Verification items for the finished model (mm, model axes). A direction names the side the tool comes from. Round coordinates to 2 decimals unless told otherwise and drop trailing zeros. Loops run counter-clockwise (first coordinate to the right, second up) from the corner with the lowest first, then second, coordinate; pieces in that order, holes last. Notation, with made-up numbers: M 69,-9 L 80,-9 A13 cw 80,14 Z; hole C 14,58 d11. An arc over 180 degrees is marked long. One line per item, written item: value.
from build123d import *

# Parameters (mm, degrees)
SKETCH1_W                        = 12
SKETCH1_H                        = 1.5
BOSS_EXTRUDE1_DEPTH              = 3
BOSS_EXTRUDE2_DEPTH              = 3
BOSS_EXTRUDE3_DEPTH              = 3
BOSS_EXTRUDE3_DEPTH_BACK         = 6
F_97_0_0059_DIAMETER_HOLE1_D     = 7.200000078
F_97_0_0059_DIAMETER_HOLE1_DEPTH = 10


with BuildPart() as part:
    # Sketch1 → Boss-Extrude1 (new body)
    with BuildSketch(Plane(origin=(0, 0, 0), x_dir=(1, 0, 0), z_dir=(0, 1, 0))):
        with Locations((6, 0.75)):
            Rectangle(SKETCH1_W, SKETCH1_H)
    extrude(amount=BOSS_EXTRUDE1_DEPTH)

    # Sketch2 → Boss-Extrude2 (add)
    with BuildSketch(Plane(origin=(0, 3, 0), x_dir=(1, 0, 0), z_dir=(0, 1, 0))):
        Polygon((0, 1.5), (-11.766968108, -0.853393621), (-11.472793906, -2.324264634), (0.294174203, 0.029128986), align=None)
    extrude(amount=-BOSS_EXTRUDE2_DEPTH)

    # Sketch4 → Boss-Extrude3 (add, two sides: drawn at the far end of the back side and taken through both)
    with BuildSketch(Plane(origin=(0, 3, 0), x_dir=(1, 0, 0), z_dir=(0, 1, 0)).offset(-BOSS_EXTRUDE3_DEPTH_BACK)):
        Polygon((-11.766968108, -0.853393621), (-9.903864825, -10.16891004), (-17.748510231, -11.737839121), (-19.611613514, -2.422322701), align=None)
    extrude(amount=BOSS_EXTRUDE3_DEPTH + BOSS_EXTRUDE3_DEPTH_BACK)

    # #97 (0.0059) Diameter Hole1
    with Locations(Plane(origin=(-19.323151976, 0, 3.864630394), x_dir=(0.19611613506937434, 0, 0.9805806757046821), z_dir=(-0.9805806757046821, 0, 0.19611613506937434))):
        with Locations((4.029128986, 1.5)):
            Hole(F_97_0_0059_DIAMETER_HOLE1_D / 2, depth=F_97_0_0059_DIAMETER_HOLE1_DEPTH)


solid = part.part
(1) Sectioned sample at B-B on z = 1.25. Enter the section's corners in (x, y).
Completed:
outline: M -13.75,-3 L -11.69,-3 L -11.69,0 L -6.1,0 L -6.1,3 L -11.69,3 L -11.69,6 L -13.75,6 Z
(2) Thickness scan on L1, parallel to Z at x = 6.5, y = 2.5; L2, parallel to Z at x = -13.5, y = -1; L3, parallel to Z at x = -12.5, y = -2.25. Record the ranges inside material, lowest first. Write a range as from..to.
Completed:
L1: z = -1.5..0
L2: z = 1.2..4.17, 9.45..10.89
L3: z = 1..10.69
(3) Depth check by flat-ended pin: pin 1 Ø4 at (y, z) = (5, 5.5) entering from -X; pin 2 Ø3.5 at (x, y) = (8, 2) entering from +Z; pin 3 Ø4 at (x, z) = (5, 1) entering from +Y. Enter the tip coordinate at first touch or a pass-through.
Completed:
pin 1: stops at x = -19.4
pin 2: stops at z = 0
pin 3: stops at y = 3
(4) Sectioned sample at C-C on x = 2.5. Enter the section's corners in (y, z).
Completed:
outline: M 0,-1.5 L 3,-1.5 L 3,0 L 0,0 Z
(5) Sectioned sample at D-D on y = 2.5. Enter the section's corners in (x, z).
Completed:
outline: M -19.61,2.42 L 0,-1.5 L 12,-1.5 L 12,0 L 0.15,0 L -11.47,2.32 L -11.37,2.86 L -19.21,4.42 Z; M -17.85,11.21 L -10.01,9.64 L -9.9,10.17 L -17.75,11.74 Z
(6) Tool access check on faces 1 (the face through (6, 1, 0)), 2 (the face through (-19.29, 1.44, 4.04)). Record the directions out of +Z, -Z, +X, -X, +Y, -Y that give a thin tool (end or side, any length) a straight path to the whole face; none if there is none.
Completed:
face 1: +Z, +X, +Y, -Y
face 2: +Z, -X, +Y, -Y
(7) Sectioned sample at A-A on y = -1.75. Enter the section's corners in (x, z).
Completed:
outline: M -19.61,2.42 L -11.77,0.85 L -10.99,4.73 L -18.84,6.3 Z; M -18.23,9.33 L -10.38,7.76 L -9.9,10.17 L -17.75,11.74 Z
(8) Mould release check, pull along Z, two halves, no side actions. Record for faces 3 (the face through (6, 1, -1.5)), 4 (the face through (12, 1, -1)), 5 (the face through (-14.882, -1.694, 5.391)), 6 (the face through (-13.771, 1.437, 10.942)): +Z half, -Z half, draft (parallel to the pull), parting line (faces both ways), or undercut.
Completed:
face 3: -Z half
face 4: draft
face 5: undercut
face 6: +Z half
